Study the drawing (mm; zero at the part's minimum x, y, z) and answer. A direction names the side the tool comes from. Coordinates: 2 decimals unless noted, no trailing zeros. Order: outer loops, then holes, each group sorted by start corner. A loop starts at its lowest first (then second) coordinate and runs counter-clockwise, first axis right, second up.
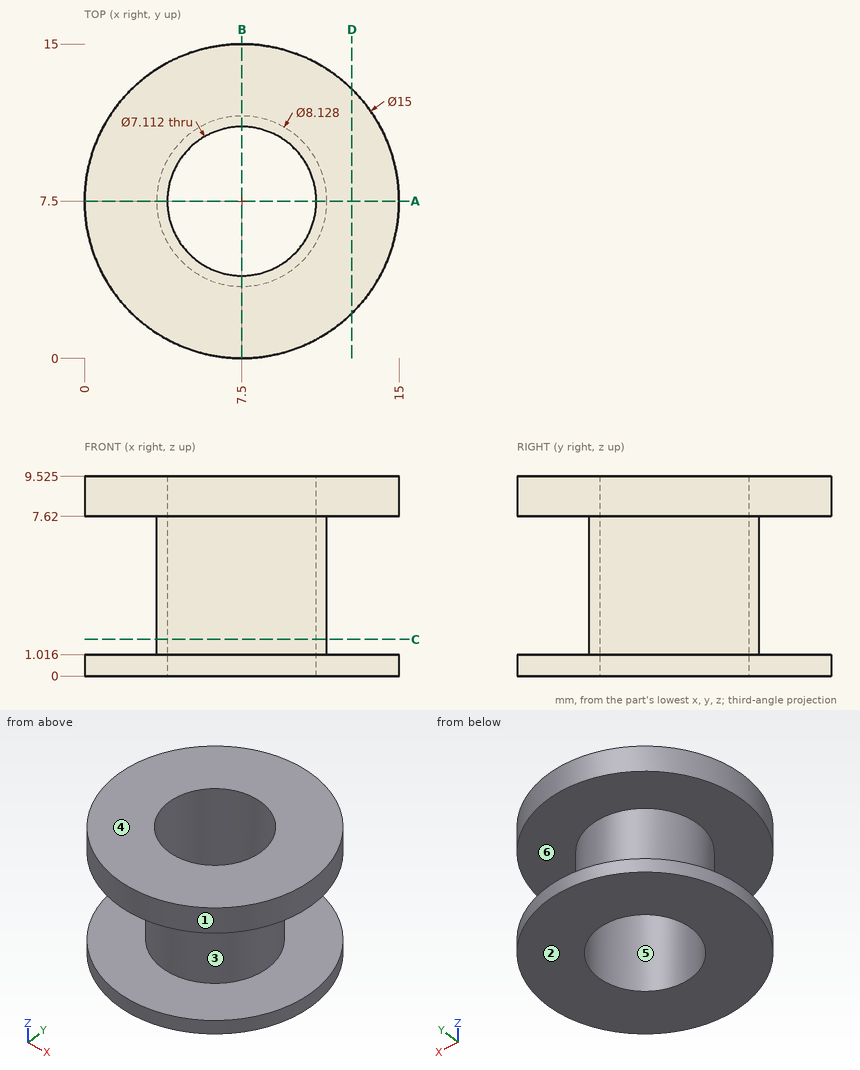
1) A cutting plane is placed at C-C, the plane z = 1.75. Determine the outline of the cut face in (x, y).
A:
outline: circle Ø8.13 at (7.5, 7.5); hole circle Ø7.11 at (7.5, 7.5)
2) A cutting plane is placed at D-D, the plane x = 12.75. Determine the outline of the cut face in (y, z) (3 decimals).
A:
outline: (2.144, 0) - (12.856, 0) - (12.856, 1.016) - (2.144, 1.016) - close; (2.144, 7.62) - (12.856, 7.62) - (12.856, 9.525) - (2.144, 9.525) - close
3) A cutting plane is placed at A-A, the plane y = 7.5. Determine the outline of the cut face in (x, z) (3 decimals).
A:
outline: (0, 0) - (3.944, 0) - (3.944, 9.525) - (0, 9.525) - (0, 7.62) - (3.436, 7.62) - (3.436, 1.016) - (0, 1.016) - close; (11.056, 0) - (15, 0) - (15, 1.016) - (11.564, 1.016) - (11.564, 7.62) - (15, 7.62) - (15, 9.525) - (11.056, 9.525) - close
4) Determine the mould class of the marked faces 1, 2, 3 and 4 for opening direction Z: pulls with the +Z half, pulls with the -Z half, needs draft (parallel to the pull), parting line crosses it, or undercut.
A:
face 1: needs draft
face 2: pulls with the -Z half
face 3: undercut
face 4: pulls with the +Z half
5) Flat-ended cylindrical pins translate along their axes: pin 1 Ø1.5 at (x, z) = (6, 8.5) entering from -Y; pin 2 Ø5 at (y, z) = (10.5, 6.5) entering from -X; pin 3 Ø4.5 at (x, y) = (8, 10.5) entering from +Z (3 decimals); pin 4 Ø2 at (y, z) = (8, 4.5) entering from -X. Find the tip coordinate at first contact, or state that the pin passes through.
A:
pin 1: stops at y = 0.04
pin 2: stops at x = 0.04
pin 3: stops at z = 9.525
pin 4: stops at x = 3.44
6) Straight lines are drawn through the part: line 1 (Y direction, x = 7.5, z = 7.25); line 2 (Z direction, x = 12.25, y = 11) (3 decimals); line 3 (Y direction, x = 6.25, z = 1.5). For each, find the intervals that lie inside material, in ascending order.
A:
line 1: y = 3.44 to 3.94, 11.06 to 11.56
line 2: z = 0 to 1.016, 7.62 to 9.525
line 3: y = 3.63 to 4.17, 10.83 to 11.37
7) Which of the six approach directions +Z, -Z, +X, -X, +Y, -Y give full straight-line access (tool end or side, diameter ignored) to the marked faces 5 and 6?
A:
face 5: +Z, -Z
face 6: none
